Autodesk Inventor part; units mm, degrees
ref_plane "YZ Plane" through (0, 0, 0) normal (1, 0, 0) x (0, 1, 0)
ref_plane "XZ Plane" through (0, 0, 0) normal (0, 1, 0) x (-1, 0, 0)
ref_plane "XY Plane" through (0, 0, 0) normal (0, 0, 1) x (1, 0, 0)
sketch "Sketch1" plane through (0, 0, 0) normal (0, 0, 1) x (1, 0, 0)
  line L0 (-22.5, -22.5) -> (22.5, -22.5)
  line L1 (22.5, -22.5) -> (22.5, 22.5)
  line L2 (22.5, 22.5) -> (-22.5, 22.5)
  line L3 (-22.5, 22.5) -> (-22.5, -22.5)
  line L4 (-22.5, -22.5) -> (22.5, 22.5) construction
  line L5 (22.5, -22.5) -> (-22.5, 22.5) construction
  circle A0 centre (0, 0) radius 11
  line L6 (0, 0) -> (0, 17)
  line L7 (0, 0) -> (15.6, -9.0067)
  line L8 (0, 0) -> (-15.6, -9.0067)
  circle A1 centre (0, 17) radius 2.6
  circle A2 centre (15.6, -9.0067) radius 2.6
  circle A3 centre (-15.6, -9.0067) radius 2.6
  point P0 (22.5, -11.0947)
  point P1 (-22.5, -11.0947)
  dimension "d0" = 45
  dimension "d1" = 45
  dimension "d2" = 22
  dimension "d3" = 17
  dimension "d4" = 15.6
  dimension "d5" = 120
  dimension "d6" = 15.6
  dimension "d7" = 120
  dimension "d8" = 5.2
  dimension "d9" = 5.2
  dimension "d10" = 5.2
extrude "Extrusion2" add sketch "Sketch1" against normal blind 3
sketch "Sketch13" plane through (0, 0, 0) normal (0, 0, 1) x (1, 0, 0)
  line L0 (0, 0) -> (0, -32)
  line L1 (-22.5, -22.5) -> (22.5, -22.5)
  line L2 (-22.5, -22.5) -> (-22.5, 22.5)
  line L3 (-22.5, -22.5) -> (22.5, -22.5)
  line L4 (22.5, -22.5) -> (22.5, -32)
  line L5 (22.5, -32) -> (-22.5, -32)
  line L6 (-22.5, -32) -> (-22.5, -22.5)
  point P0 (22.5, -22.5)
  dimension "d28" = 32
extrude "Extrusion6" add sketch "Sketch13" against normal blind 20
sketch "Sketch14" plane through (-22.5, -22.5, -3) normal (0, 1, 0) x (1, 0, 0)
  line L0 (45, 0) -> (0, 0)
  line L1 (45, 0) -> (45, 17)
  line L2 (0, 17) -> (45, 17)
  line L3 (0, 0) -> (0, 17)
  circle A0 centre (22.5, 8.5) radius 3
  point P0 (22.5, -3)
  dimension "d31" = 6
sketch "Sketch15" plane through (-22.5, -22.5, -3) normal (0, 1, 0) x (1, 0, 0)
  circle A0 centre (22.5, 8.4604) radius 5
  point P0 (22.5, -3)
  dimension "d32" = 10
extrude "Extrusion7" cut sketch "Sketch14" against normal blind 10 contours A0
extrude "Extrusion8" cut sketch "Sketch15" against normal blind 6
equation "\"d1\" = d0"
equation "\"d4\" = d6"
equation "\"d7\" = d5"
equation "\"d9\" = d8"
equation "\"d10\" = d8"
properties part number "mount_v10"
Verification items for the finished model (mm, model axes). A direction names the side the tool comes from. Round coordinates to 2 decimals unless told otherwise and drop trailing zeros. Loops run counter-clockwise (first coordinate to the right, second up) from the corner with the lowest first, then second, coordinate; pieces in that order, holes last. Notation, with made-up numbers: (19, 20.25) - (61, 20.25) arc R18 ccw to (61, 46.25) - close; hole circle Ø2 at (28.5, -36). An arc over 180 degrees is marked (long way). Use a Markdown table: item, result. Add a question column.
1. Section check B-B, the plane x = 0. Record the boundary of the cut face in (y, z), plus the area to 3 significant figures.
2. Access from +Z, -Z, +X, -X, +Y, -Y to the whole of each face (thin tool, end or side, straight path). Record for faces 1 (the face through (-5.3, -22.5, -11.4)), 2 (the face through (22.5, -15, -2.5)).
3. Section check D-D, the plane x = -15.6. Record the boundary of the cut face in (y, z).
4. Gauge pin test, flat ends, axial feed: pin 1 (5 mm diameter, centred on x = 0.5, z = -10.5, fed in from +Y); pin 2 (22.5 mm diameter, centred on x = -11, y = -0.5, fed in from -Z); pin 3 (5 mm diameter, centred on x = 8, z = -15.5, fed in from +Y). Record the tip position at first contact, or that the pin passes through.
5. Section check C-C, the plane z = -13.75. Record the boundary of the cut face in (x, y).
6. Release check for a two-part mould opening along Z. For faces 3 (the face through (-5, -10, 0)), 4 (the face through (2, -28.5, -9)), 5 (the face through (-14.4, -11.313, -1.479)), 6 (the face through (-1.08, -25.46, -6.58)) record: released by +Z, released by -Z, zero draft, split by the parting line, or undercut.
7. Section check A-A, the plane y = 17. Record the boundary of the cut face in (x, z), plus the area to 3 significant figures.
8. Thickness scan on probe 1 along Y at (x, z) = (0, -1.45); probe 2 along X at (y, z) = (17, -0.9); probe 3 along Z at (x, y) = (0, -30.65). Record the ranges inside material, lowest first. Write a range as [from, to].
Checks:
| question | item | result |
|---|---|---|
| 1 | outline | (-32, -20) - (-22.5, -20) - (-22.5, -16.46) - (-28.5, -16.46) - (-28.5, -14.5) - (-32, -14.5) - close; (-32, -8.5) - (-28.5, -8.5) - (-28.5, -6.46) - (-22.5, -6.46) - (-22.5, -3) - (-11, -3) - (-11, 0) - (-32, 0) - close; (11, -3) - (14.4, -3) - (14.4, 0) - (11, 0) - close; (19.6, -3) - (22.5, -3) - (22.5, 0) - (19.6, 0) - close |
| 1 | area | 162 mm^2 |
| 2 | face 1 | -Z, +X, -X, +Y |
| 2 | face 2 | +Z, -Z, +X, +Y, -Y |
| 3 | outline | (-32, -20) - (-22.5, -20) - (-22.5, -3) - (-11.61, -3) - (-11.61, 0) - (-32, 0) - close; (-6.41, -3) - (22.5, -3) - (22.5, 0) - (-6.41, 0) - close |
| 4 | pin 1 | stops at y = -28.5 |
| 4 | pin 2 | stops at z = -3 |
| 4 | pin 3 | stops at y = -22.5 |
| 5 | outline | (-22.5, -32) - (-1.98, -32) - (-1.98, -28.5) - (-4.44, -28.5) - (-4.44, -22.5) - (-22.5, -22.5) - close; (1.98, -32) - (22.5, -32) - (22.5, -22.5) - (4.44, -22.5) - (4.44, -28.5) - (1.98, -28.5) - close |
| 6 | face 3 | released by +Z |
| 6 | face 4 | undercut |
| 6 | face 5 | zero draft |
| 6 | face 6 | undercut |
| 7 | outline | (-22.5, -3) - (-2.6, -3) - (-2.6, 0) - (-22.5, 0) - close; (2.6, -3) - (22.5, -3) - (22.5, 0) - (2.6, 0) - close |
| 7 | area | 119 mm^2 |
| 8 | probe 1 | y = [-32, -11], [11, 14.4], [19.6, 22.5] |
| 8 | probe 2 | x = [-22.5, -2.6], [2.6, 22.5] |
| 8 | probe 3 | z = [-20, -14.5], [-8.5, 0] |
